Could you check a few things on this model? Use its own coordinates, in mm. A direction names the side the tool comes from. Coordinates: 2 decimals unless noted, no trailing zeros. Loops run counter-clockwise (first coordinate to the right, second up) from the corner with the lowest first, then second, coordinate; pieces in that order, holes last. Notation, with made-up numbers: (89.25, 8.25) - (109.25, 8.25) arc R15 ccw to (109.25, 35.25) - close; hole circle Ø3 at (-6.5, 57). An arc over 180 degrees is marked (long way). One line per item, written item: value. Start each with the question number.
(1) If we section it at A-A on y = 37: Write out the boundary of the cut face in (x, z).
(2) If I drill on line 1 along X through (y, z) = (33, 37); line 2 along X through (y, z) = (41, 10.5); line 3 along Z through (x, y) = (37.5, 20), over which ranges is the centre line in solid material (lowest first)? Write a range as from..to.
(3) If we section it at C-C on x = 37.5: Write out the boundary of the cut face in (y, z).
(4) On a 3-axis mill with a long thin cutter (end or side, diameter ignored), from which of +Z, -Z, +X, -X, +Y, -Y can I reach the whole of each face in a straight line? I mean faces 4 (the face through (35, 30, 35)), 5 (the face through (45, 30, 0)). Say none if no direction works.
(5) If we mould it in two halves opening along X, with no side actions, what happens to faces 1 (the face through (25, 30, 15)), 2 (the face through (0, 30, 20)), 3 (the face through (43, 30, 40))? For each: pulls with the +X half, pulls with the -X half, needs draft (parallel to the pull), parting line crosses it, or undercut.
(6) I'm going to push flat-ended pins straight in: P1, Ø3, axis at y = 24.5, z = 37, coming from the -X side; P2, Ø10, axis at x = 29, y = 16, coming from the +Z side; P3, Ø12, axis at x = 21.5, y = 8, coming from the -Z side. Where does each tip first touch, or does it pass through?
(7) If we section it at B-B on x = 25: Write out the boundary of the cut face in (y, z).
```python
from build123d import *

# Parameters (mm, degrees)
F1_DEPTH = 60


with BuildPart() as f1:
    # F0 (on Front) → F1 (new body)
    with BuildSketch(Plane.XZ):
        with BuildLine():
            Line((0, 40), (0, 0))
            Line((0, 0), (10, 0))
            ThreePointArc((10, 0), (25, 15), (40, 0))
            Line((40, 0), (50, 0))
            Line((50, 0), (50, 40))
            Line((50, 40), (35, 40))
            Line((35, 40), (35, 30))
            Line((35, 30), (15, 30))
            Line((15, 30), (15, 40))
            Line((15, 40), (0, 40))
        make_face()
    extrude(amount=-F1_DEPTH)


solid = f1.part
```
Values:
1. outline: (0, 0) - (10, 0) arc R15 cw to (40, 0) - (50, 0) - (50, 40) - (35, 40) - (35, 30) - (15, 30) - (15, 40) - (0, 40) - close
2. line 1: x = 0..15, 35..50
2. line 2: x = 0..14.29, 35.71..50
2. line 3: z = 8.29..40
3. outline: (0, 8.29) - (60, 8.29) - (60, 40) - (0, 40) - close
4. face 4: +Z, +Y, -Y
4. face 5: -Z, +X, -X, +Y, -Y
5. face 1: undercut
5. face 2: pulls with the -X half
5. face 3: needs draft
6. P1: stops at x = 0
6. P2: stops at z = 30
6. P3: stops at z = 11.61
7. outline: (0, 15) - (60, 15) - (60, 30) - (0, 30) - close
